Input: part model. Units: mm. Frame: model coordinates. A direction names the side the tool comes from. Coordinates: 2 decimals unless noted, no trailing zeros. Order: outer loops, then holes, each group sorted by start corner. A loop starts at its lowest first (then second) coordinate and runs counter-clockwise, first axis right, second up. Notation, with made-up numbers: (12, -14.75) - (52, -14.75) arc R21 ccw to (52, -8.75) - close; hole circle Ø8 at (11, 65.5). An arc over 180 degrees is marked (long way). Use a Markdown table: item, result. Add a question column.
from build123d import *

# Parameters (mm, degrees)
SKETCH1_R           = 105
SKETCH1_R_2         = 100
BOSS_EXTRUDE3_DEPTH = 100
SKETCH2_W           = 48.620736816
SKETCH2_H           = 22.255971078
CUT_EXTRUDE2_DEPTH  = 187


with BuildPart() as part:
    # Sketch1 → Boss-Extrude3 (new body)
    with BuildSketch(Plane(origin=(0, 0, 0), x_dir=(1, 0, 0), z_dir=(0, 1, 0))):
        Circle(SKETCH1_R)
        Circle(SKETCH1_R_2, mode=Mode.SUBTRACT)
    extrude(amount=BOSS_EXTRUDE3_DEPTH)

    # Sketch2 → Cut-Extrude2 (cut)
    with BuildSketch(Plane.XY):
        with Locations((0, 50)):
            Rectangle(SKETCH2_W, SKETCH2_H)
    extrude(amount=-CUT_EXTRUDE2_DEPTH, mode=Mode.SUBTRACT)


solid = part.part
1) Cut plane A-A (z = 0). Return the cut outline in (x, y).
2) Cut plane B-B (x = 0). Return the cut outline in (y, z), and give its area (3 significant figures).
3) Cut plane C-C (x = 48.5). Return the cut outline in (y, z).
4) Reachability of faces 4 (the flat face through (93, 0, 38)), 5 (the flat face through (-24.31, 50, -100)) from +Z, -Z, +X, -X, +Y, -Y: full face, straight path, thin tool, end or side. Return the list, or none.
5) Material intervals for L1, parallel to Z at x = 0, y = 34; L2, parallel to Z at x = 30, y = 85.5, sorted ascending.
6) Cut plane D-D (y = 69.5). Return the cut outline in (x, z).
7) Contact query for flat-ended pins moving along their axis: P1, Ø2, axis at x = 69, y = 21, coming from the -Z side; P2, Ø4, axis at y = 46, z = -99, coming from the -X side; P3, Ø2, axis at x = 36.5, y = 17.5, coming from the -Z side. Output: stop coordinate, or through.
8) Pull-direction query (X, two-part tool) for faces 1 (the cylindrical face through (-22.762, 49.3, 102.503)), 2 (the flat face through (0, 61.128, -102)), 3 (the flat face through (93, 100, 38)); classes: pulls with the +X half, pulls with the -X half, needs draft (parallel to the pull), parting line crosses it, or undercut.
Computed:
| question | item | result |
|---|---|---|
| 1 | outline | (-105, 0) - (-100, 0) - (-100, 100) - (-105, 100) - close; (100, 0) - (105, 0) - (105, 100) - (100, 100) - close |
| 2 | outline | (0, -105) - (38.87, -105) - (38.87, -100) - (0, -100) - close; (0, 100) - (100, 100) - (100, 105) - (0, 105) - close; (61.13, -105) - (100, -105) - (100, -100) - (61.13, -100) - close |
| 2 | area | 889 mm2 |
| 3 | outline | (0, -93.13) - (100, -93.13) - (100, -87.45) - (0, -87.45) - close; (0, 87.45) - (100, 87.45) - (100, 93.13) - (0, 93.13) - close |
| 4 | face 4 | +Z, -Z, +X, -X, -Y |
| 4 | face 5 | -Z |
| 5 | L1 | z = -105 to -100, 100 to 105 |
| 5 | L2 | z = -100.62 to -95.39, 95.39 to 100.62 |
| 6 | outline | circle Ø210 at (0, 0); hole circle Ø200 at (0, 0) |
| 7 | P1 | stops at z = -80.01 |
| 7 | P2 | stops at x = -40.2 |
| 7 | P3 | stops at z = -98.82 |
| 8 | face 1 | parting line crosses it |
| 8 | face 2 | undercut |
| 8 | face 3 | needs draft |
